Study the drawing (mm; zero at the part's minimum x, y, z) and answer. Coordinates: 2 decimals unless noted, no trailing zeros. Loops run counter-clockwise (first coordinate to the right, second up) from the corner with the lowest first, then second, coordinate; pieces in that order, holes last.
Q1. Section D-D (z = 240) is taken. Give the vertices of the cut face in (x, y), then the cut area to 3 significant figures.
Q2. Straight lines are drawn through the part: line 1 (X direction, y = 13.5, z = 95); line 2 (Z direction, x = 40, y = 9.5); line 3 (Z direction, x = 26, y = 16.75). For each, find the intervals that lie inside material, in ascending order.
Q3. The mould has two halves that part along Z. Classify the marked faces 1, 2 and 3: pulls with the +Z half, pulls with the -Z half, needs draft (parallel to the pull), parting line crosses it, or undercut.
Q4. Section A-A (x = 71) is taken. Give the vertices of the cut face in (y, z).
Q5. Section C-C (x = 40) is taken. Give the vertices of the cut face in (y, z), then the cut area to 3 significant figures.
Q6. Section B-B (z = 15) is taken. Give the vertices of the cut face in (x, y).
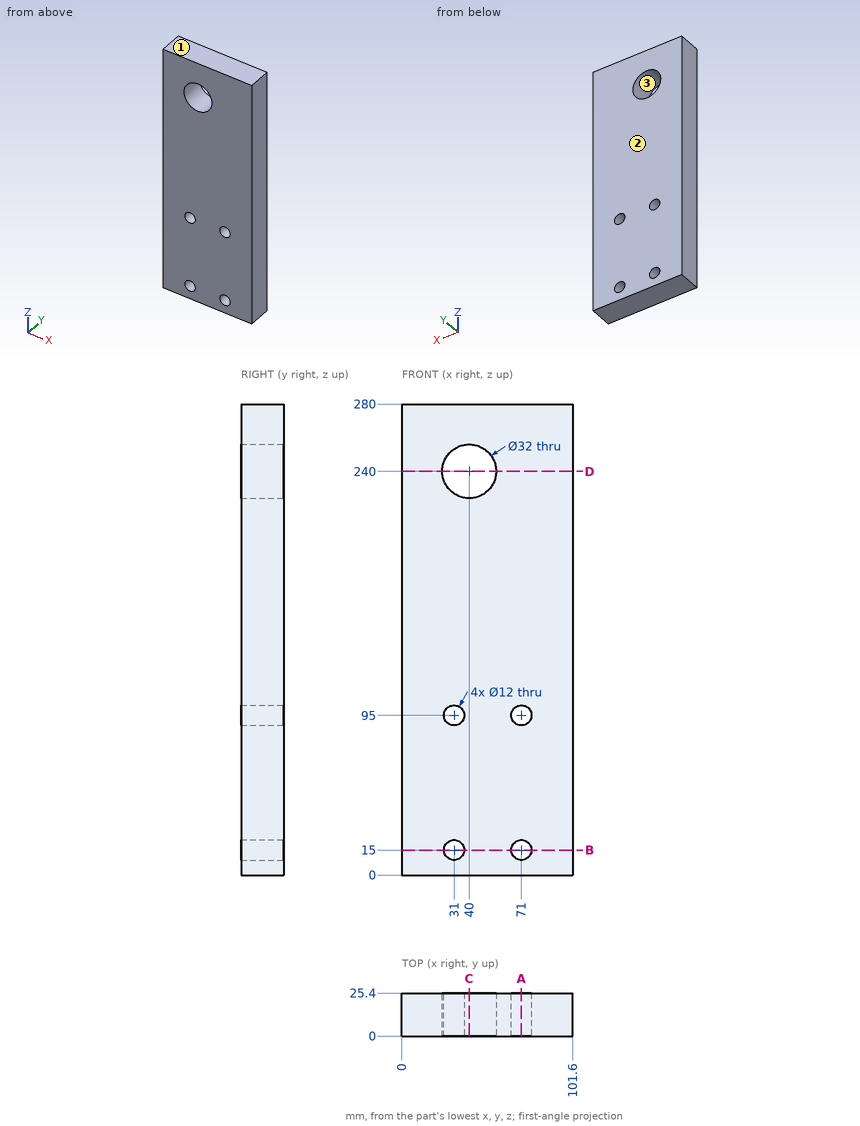
Numbers:
1. outline: (0, 0) - (24, 0) - (24, 25.4) - (0, 25.4) - close; (56, 0) - (101.6, 0) - (101.6, 25.4) - (56, 25.4) - close
1. area: 1,770 mm2
2. line 1: x = 0 to 25, 37 to 65, 77 to 101.6
2. line 2: z = 0 to 224, 256 to 280
2. line 3: z = 0 to 11.68, 18.32 to 91.68, 98.32 to 232.25, 247.75 to 280
3. face 1: pulls with the +Z half
3. face 2: needs draft
3. face 3: undercut
4. outline: (0, 0) - (25.4, 0) - (25.4, 9) - (0, 9) - close; (0, 21) - (25.4, 21) - (25.4, 89) - (0, 89) - close; (0, 101) - (25.4, 101) - (25.4, 280) - (0, 280) - close
5. outline: (0, 0) - (25.4, 0) - (25.4, 224) - (0, 224) - close; (0, 256) - (25.4, 256) - (25.4, 280) - (0, 280) - close
5. area: 6,300 mm2
6. outline: (0, 0) - (25, 0) - (25, 25.4) - (0, 25.4) - close; (37, 0) - (65, 0) - (65, 25.4) - (37, 25.4) - close; (77, 0) - (101.6, 0) - (101.6, 25.4) - (77, 25.4) - close
